Read the model definition and answer for the solid it produces. Units are mm, in the model's axes. A direction names the side the tool comes from. Give positions to 0.01 mm unless a question says otherwise; leave off trailing zeros. Write each loop counter-clockwise with the first axis right and the second up, starting at its lowest first coordinate (ties: lowest second). Pieces come first, ordered by that corner, then holes. Notation, with made-up numbers: (87, -35.75) - (140, -35.75) arc R17 ccw to (140, -4.75) - close; hole circle Ø4 at (15.25, 14.5). An arc over 180 degrees is marked (long way). Use CSV: the item, a comma, the result in double quotes. Start each with the question number.
from build123d import *

# Parameters (mm, degrees)
F2_R = 5.08
F3_R = 50.8


with BuildPart() as f1:
    # F0 (on Front) → F1 (revolve)
    with BuildSketch(Plane.XZ):
        Polygon((15.24, 120.65), (0, 120.65), (0, -120.65), (31.75, -120.65), (31.75, -19.05), (15.24, 28.955315), align=None)
    revolve(axis=Axis((0, 0, 2.313137), (0, 0, -1)))

    # F2
    f2_edges = [f1.edges().sort_by_distance(p)[0] for p in [
        (-31.75, 0, -120.65),
    ]]
    fillet(f2_edges, radius=F2_R)

    # F3
    f3_edges = [f1.edges().sort_by_distance(p)[0] for p in [
        (-31.75, 0, -19.05),
        (-15.24, 0, 28.955315),
    ]]
    fillet(f3_edges, radius=F3_R)


solid = f1.part
(1) Which of the six approach directions +Z, -Z, +X, -X, +Y, -Y give full straight-line access (tool end or side, diameter ignored) to faces 1 (the face through (0, 0, 120.65)), 2 (the face through (-3.3, 14.88, 79.63))?
(2) The part is cut by section A-A on z = 87.5. Write down the section's boundary in (x, y).
(3) The part is cut by section B-B on z = 12. Write down the section's boundary in (x, y).
(4) Given P1, Ø1, axis at x = 12.5, z = -55, coming from the +Y side; P2, Ø10, axis at x = -5, z = 1.5, coming from the +Y side; P3, Ø8, axis at x = 15.5, z = 82.5, coming from the -Y side; P4, Ø10, axis at y = 25, z = 78, coming from the -X side, each flat-ended and moving along its own axis, determine where each tip first touches the part or whether it passes through.
(5) Consider probe 1 along X at (y, z) = (-1, 62); probe 2 along Y at (x, z) = (22, -52); probe 3 along X at (y, z) = (-24, -51). Determine where each line is inside the solid, lowest interval first.
Reported:
1,face 1,"+Z, +X, -X, +Y, -Y"
1,face 2,"+Z"
2,outline,"circle Ø30.48 at (0, 0)"
3,outline,"circle Ø42.14 at (0, 0)"
4,P1,"y = 29.39"
4,P2,"y = 26.09"
4,P3,"y = -10"
4,P4,"through"
5,probe 1,"-15.21 to 15.21"
5,probe 2,"-22.89 to 22.89"
5,probe 3,"-20.79 to 20.79"
